The listing builds one solid part. Answer for the finished solid, in the listing's coordinates (mm). Face numbers are marked on the shaded views. A direction names the side the tool comes from. Give positions to 0.01 mm unless a question says otherwise; leave off trailing zeros. Loops run counter-clockwise (first coordinate to the right, second up) from the corner with the lowest first, then second, coordinate; pieces in that order, holes last. Notation, with made-up numbers: M 34.25,10.25 L 48.25,10.25 A13 cw 48.25,20.25 Z; hole C 8,21.25 d10. An arc over 180 degrees is marked long. Use one line per item in the form item = value. Start each with the question number.
1. For the marked faces 1, 2 and 3, determine the directions among +Z, -Z, +X, -X, +Y, -Y from which every point of the face is accessible in a straight line to the end or side of a thin tool.
2. The part is cut by section D-D (x = 17). Write down the section's boundary in (y, z).
3. The mould has two halves that part along X. Classify the marked faces 4, 5, 6 and 7: released by +X, released by -X, zero draft, split by the parting line, or undercut.
4. Straight lines are drawn through the part: line 1 (X direction, y = -6, z = 9); line 2 (Z direction, x = -6, y = -2.25); line 3 (X direction, y = -0.75, z = -1.5). For each, find the intervals that lie inside material, in ascending order. Write a range as from..to.
5. The part is cut by section A-A (y = 0). Write down the section's boundary in (x, z), and give its area (3 significant figures).
6. The part is cut by section B-B (z = 9.5). Write down the section's boundary in (x, y), and give its area (3 significant figures).
7. The part is cut by section C-C (x = -11). Write down the section's boundary in (y, z), and give its area (3 significant figures).
8. Each of these flat-tipped pins is pushed along its axis until it touches: pin 1 Ø3 at (y, z) = (4.5, 9.5) entering from -X; pin 2 Ø10 at (x, y) = (1.5, -3) entering from -Z; pin 3 Ø4 at (x, y) = (10, 0) entering from +Z; pin 4 Ø1 at (x, z) = (-7.5, -1) entering from -Y. Where does it stop, or does it pass through?
from build123d import *

# Parameters (mm, degrees)
SCHIZZO1_W                   = 48
SCHIZZO1_H                   = 20
ESTRUSIONE_ESTRUSIONE1_DEPTH = 5
SCHIZZO2_W                   = 3
SCHIZZO2_H                   = 20
SCHIZZO2_W_2                 = 10
ESTRUSIONE_ESTRUSIONE2_DEPTH = 25
TAGLIO_ESTRUSIONE1_REACH     = 59.48
SCHIZZO3_R                   = 21.2
SCHIZZO4_R                   = 2.5
ESTRUSIONE_ESTRUSIONE3_DEPTH = 5


with BuildPart() as part:
    # Schizzo1 → Estrusione-Estrusione1 (new body)
    with BuildSketch(Plane.XY):
        Rectangle(SCHIZZO1_W, SCHIZZO1_H)
    extrude(amount=ESTRUSIONE_ESTRUSIONE1_DEPTH)

    # Schizzo2 → Estrusione-Estrusione2 (add)
    with BuildSketch(Plane.XY.offset(5)):
        with Locations((-22.5, 0)):
            Rectangle(SCHIZZO2_W, SCHIZZO2_H)
        with Locations((19, 0)):
            Rectangle(SCHIZZO2_W_2, SCHIZZO2_H)
    extrude(amount=ESTRUSIONE_ESTRUSIONE2_DEPTH)

    # Taglio-Estrusione1: up to this face of the body (flat: up to its plane)
    taglio_estrusione1_end = Plane(part.part.faces().sort_by_distance((24, 0, 15))[0])
    # Schizzo3 → Taglio-Estrusione1 (cut, up to the picked face)
    with BuildSketch(Plane.ZY.offset(24), mode=Mode.PRIVATE) as taglio_estrusione1_sk1:
        with Locations((30, 0)):
            Circle(SCHIZZO3_R)
    taglio_estrusione1_tool1 = split(extrude(taglio_estrusione1_sk1.sketch, amount=-TAGLIO_ESTRUSIONE1_REACH, mode=Mode.PRIVATE), bisect_by=taglio_estrusione1_end, keep=Keep.BOTH, mode=Mode.PRIVATE)
    add(taglio_estrusione1_tool1.solids().sort_by(Axis((-24, 0, 30), (1, 0, 0)))[0], mode=Mode.SUBTRACT)

    # Schizzo4 → Estrusione-Estrusione3 (add)
    with BuildSketch(Plane(origin=(0, 0, 0), x_dir=(-1, 0, 0), z_dir=(0, 0, -1))):
        with Locations(Location((-9, 0, 0), (0, 0, 180))):
            Circle(SCHIZZO4_R)
        with Locations(Location((11, 0, 0), (0, 0, 180))):
            Circle(SCHIZZO4_R)
    extrude(amount=ESTRUSIONE_ESTRUSIONE3_DEPTH)


solid = part.part
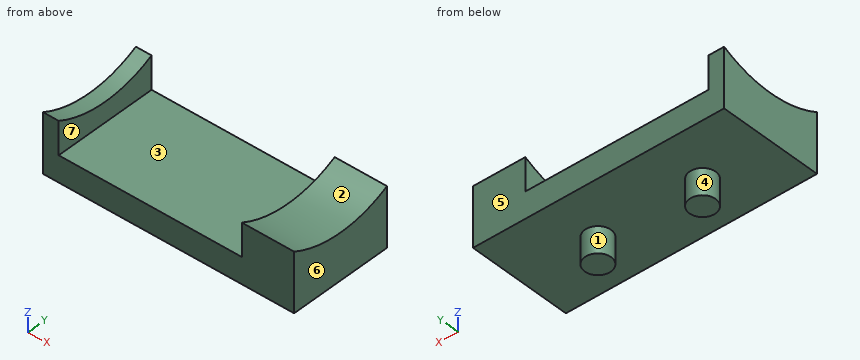
Derived:
q1.face_1 = -Z
q1.face_2 = +Z, +X, -X
q1.face_3 = +Z, +Y, -Y
q2.outline = M -10,0 L 10,0 L 10,11.31 A21.2 cw -10,11.31 Z
q3.face_4 = undercut
q3.face_5 = zero draft
q3.face_6 = released by +X
q3.face_7 = undercut
q4.line_1 = -24..-21, 14..24
q4.line_2 = 0..5
q4.line_3 = -13.38..-8.62, 6.62..11.38
q5.outline = M -24,0 L -13.5,0 L -13.5,-5 L -8.5,-5 L -8.5,0 L 6.5,0 L 6.5,-5 L 11.5,-5 L 11.5,0 L 24,0 L 24,8.8 L 14,8.8 L 14,5 L -21,5 L -21,8.8 L -24,8.8 Z
q5.area = 339 mm2
q6.outline = M -24,-10 L -21,-10 L -21,-5.4 L -24,-5.4 Z; M -24,5.4 L -21,5.4 L -21,10 L -24,10 Z; M 14,-10 L 24,-10 L 24,-5.4 L 14,-5.4 Z; M 14,5.4 L 24,5.4 L 24,10 L 14,10 Z
q6.area = 120 mm2
q7.outline = M -10,0 L -2.5,0 L -2.5,-5 L 2.5,-5 L 2.5,0 L 10,0 L 10,5 L -10,5 Z
q7.area = 125 mm2
q8.pin_1 = -24
q8.pin_2 = 0
q8.pin_3 = 5
q8.pin_4 = through
